Source: CAD feature listing. Evaluate the final solid. Frame: model axes, mm. Round coordinates to 2 decimals unless told otherwise and drop trailing zeros. Loops run counter-clockwise (first coordinate to the right, second up) from the corner with the lowest first, then second, coordinate; pieces in that order, holes last.
(1) Material intervals for probe 1 along Z at (x, y) = (0, -6.75) (3 decimals); probe 2 along Z at (x, y) = (-10.5, -2) (3 decimals); probe 3 along Z at (x, y) = (10, -2.5) (3 decimals), sorted ascending.
(2) Section C-C, the plane x = -15. Return the cut outline in (y, z) (3 decimals).
(3) Section A-A, the plane x = 0. Return the cut outline in (y, z) (3 decimals), plus the area to 3 significant figures.
(4) First-contact query: pin 1 Ø10 at (x, z) = (0, 36.9) entering from +Y. Flat tip, straight axial feed; report the tip coordinate or a pass-through.
(5) Section B-B, the plane z = 0. Return the cut outline in (x, y) (3 decimals), plus the area to 3 significant figures.
(6) Section D-D, the plane y = -6. Count the separate pieces of the cut face and the enclosed holes in it, plus the area to 3 significant figures.
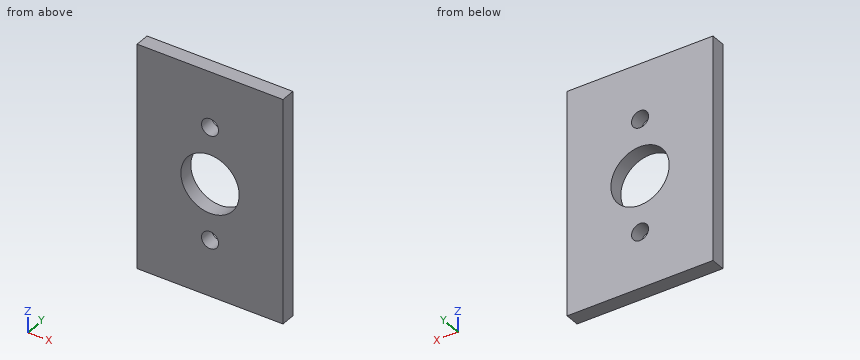
```python
from build123d import *

# Parameters (mm, degrees)
F1_W     = 95.25
F1_H     = 146.05
F2_DEPTH = 9.525
F3_D     = 38.1
F3_DEPTH = 12.7
F3_TIP   = 11.4463947925
F4_D     = 11.1125
F5_D     = 11.1125


with BuildPart() as f2:
    # F1 (on Front) → F2 (new body)
    with BuildSketch(Plane.XZ):
        Rectangle(F1_W, F1_H)
    extrude(amount=F2_DEPTH)

    # F3
    with Locations(Plane(origin=(0, 0, 0), x_dir=(1, 0, 0), z_dir=(0, 1, 0))):
        with Locations((0, 0)):
            Hole(F3_D / 2, depth=F3_DEPTH)
            with Locations((0, 0, -(F3_DEPTH + F3_TIP / 2))):  # 118° drill point
                Cone(0, F3_D / 2, F3_TIP, mode=Mode.SUBTRACT)

    # F4 (through all)
    with Locations(Plane(origin=(0, 0, 0), x_dir=(1, 0, 0), z_dir=(0, 1, 0))):
        with Locations((0, -36.9038395584)):
            Hole(F4_D / 2)

    # F5 (through all)
    with Locations(Plane(origin=(0, 0, 0), x_dir=(1, 0, 0), z_dir=(0, 1, 0))):
        with Locations((0, 36.4790037274)):
            Hole(F5_D / 2)


solid = f2.part
```
Output values:
1. probe 1: z = -73.025 to -42.035, -30.923 to -19.05, 19.05 to 31.348, 42.46 to 73.025
1. probe 2: z = -73.025 to -15.895, 15.895 to 73.025
1. probe 3: z = -73.025 to -16.214, 16.214 to 73.025
2. outline: (-9.525, -73.025) - (0, -73.025) - (0, -11.743) - (-9.525, -11.743) - close; (-9.525, 11.743) - (0, 11.743) - (0, 73.025) - (-9.525, 73.025) - close
3. outline: (-9.525, -73.025) - (0, -73.025) - (0, -42.035) - (-9.525, -42.035) - close; (-9.525, -30.923) - (0, -30.923) - (0, -19.05) - (-9.525, -19.05) - close; (-9.525, 19.05) - (0, 19.05) - (0, 31.348) - (-9.525, 31.348) - close; (-9.525, 42.46) - (0, 42.46) - (0, 73.025) - (-9.525, 73.025) - close
3. area: 817 mm2
4. pin 1: passes through
5. outline: (-47.625, -9.525) - (-19.05, -9.525) - (-19.05, 0) - (-47.625, 0) - close; (19.05, -9.525) - (47.625, -9.525) - (47.625, 0) - (19.05, 0) - close
5. area: 544 mm2
6. separate pieces: 1
6. enclosed holes: 3
6. area: 12,600 mm2
